Could you check a few things on this model? Use its own coordinates, in mm. A direction names the side the tool comes from. Give positions to 0.01 mm unless a question says otherwise; leave off trailing zeros. Loops run counter-clockwise (first coordinate to the right, second up) from the corner with the lowest first, then second, coordinate; pieces in that order, holes last. Notation, with made-up numbers: (58.25, 53) - (86.25, 53) arc R9 ccw to (86.25, 58) - close; hole circle Ø8 at (-38, 79.25). An arc over 180 degrees is marked (long way). Use CSV: the item, a comma, the result in double quotes.
Autodesk Inventor part; units mm, degrees
ref_plane "YZ Plane" through (0, 0, 0) normal (1, 0, 0) x (0, 1, 0)
ref_plane "XZ Plane" through (0, 0, 0) normal (0, 1, 0) x (-1, 0, 0)
ref_plane "XY Plane" through (0, 0, 0) normal (0, 0, 1) x (1, 0, 0)
sketch "main" plane through (0, 0, 0) normal (0, 0, 1) x (1, 0, 0)
  circle A0 centre (20.1733, 30.7236) radius 2.0955
  arc A1 (-24.2767, -13.7264) -> (-5.2267, 5.3236) centre (-24.2767, 5.3236) ccw
  line L0 (-5.2267, 14.8486) -> (-5.2267, 5.3236)
  line L1 (0.4529, -22.9162) -> (25.8529, 27.8838)
  arc A2 (-5.2267, 14.8486) -> (-14.7517, 24.3736) centre (-14.7517, 14.8486) ccw
  line L2 (-17.9267, 24.3736) -> (-14.7517, 24.3736)
  arc A3 (25.8529, 27.8838) -> (20.1733, 37.0736) centre (20.1733, 30.7236) ccw
  line L3 (20.1733, 37.0736) -> (-17.9267, 37.0736)
  line L4 (-30.6267, -13.7264) -> (-24.2767, -13.7264)
  circle A4 centre (-5.2267, -20.0764) radius 2.1844
  arc A5 (-5.2267, -26.4264) -> (0.4529, -22.9162) centre (-5.2267, -20.0764) ccw
  line L5 (-5.2267, -26.4264) -> (-30.6267, -26.4264)
  line L6 (-5.2267, -26.4264) -> (-30.6267, -26.4264)
  circle A6 centre (-30.6267, -20.0764) radius 2.1844
  arc A7 (-30.6267, -13.7264) -> (-30.6267, -26.4264) centre (-30.6267, -20.0764) ccw
  circle A8 centre (-5.2267, 30.7236) radius 2.1844
  circle A9 centre (7.4733, 5.3236) radius 2.0955
  arc A10 (-17.9267, 37.0736) -> (-17.9267, 24.3736) centre (-17.9267, 30.7236) ccw
  circle A11 centre (-17.9267, 30.7236) radius 2.1844
  point P0 (-10.623, 1.8831)
  point P1 (-5.2267, -13.7264)
  dimension "d0" = 12.7
  dimension "d1" = 12.7
  dimension "d2" = 4.3688
  dimension "d3" = 19.05
  dimension "d4" = 9.525
  dimension "d7" = 4.3688
  dimension "d8" = 4.191
  dimension "d10" = 4.191
sketch "Sketch1" plane through (0, 0, 0) normal (0, 0, 1) x (1, 0, 0)
  circle A0 centre (50.8, 0) radius 2.0955
  arc A1 (6.35, -44.45) -> (25.4, -25.4) centre (6.35, -25.4) ccw
  line L0 (25.4, -15.875) -> (25.4, -25.4)
  line L1 (31.0796, -53.6398) -> (56.4796, -2.8398)
  arc A2 (25.4, -15.875) -> (15.875, -6.35) centre (15.875, -15.875) ccw
  line L2 (12.7, -6.35) -> (15.875, -6.35)
  arc A3 (56.4796, -2.8398) -> (50.8, 6.35) centre (50.8, 0) ccw
  line L3 (50.8, 6.35) -> (12.7, 6.35)
  line L4 (0, -44.45) -> (6.35, -44.45)
  circle A4 centre (25.4, -50.8) radius 2.1844
  arc A5 (25.4, -57.15) -> (31.0796, -53.6398) centre (25.4, -50.8) ccw
  line L5 (25.4, -57.15) -> (0, -57.15)
  line L6 (25.4, -57.15) -> (0, -57.15)
  circle A6 centre (0, -50.8) radius 2.1844
  arc A7 (0, -44.45) -> (0, -57.15) centre (0, -50.8) ccw
  circle A8 centre (25.4, 0) radius 2.1844
  circle A9 centre (38.1, -25.4) radius 2.0955
  arc A10 (12.7, 6.35) -> (12.7, -6.35) centre (12.7, 0) ccw
  circle A11 centre (12.7, 0) radius 2.1844
  point P0 (0, 0)
extrude "Extrusion1" add sketch "Sketch1" along normal blind 1.5875
properties part number "gusset" material "Acetal Resin, White"
1) Which directions (+Z, -Z, +X, -X, +Y, -Y) give clear straight access to the entire face, cutting with the end or side of a thin tool? Please do faces 5 (the flat face through (25.4, -21, 1)), 6 (the flat face through (32, 6.35, 1)).
Answer below:
face 5,"+Z, -Z, -X"
face 6,"+Z, -Z, +X, -X, +Y"
2) We'd pull the mould along Y, two halves only. Please class faces 1 (the cylindrical face through (6.35, -0.14, 0.78)), 2 (the flat face through (13, -57.15, 1)), 3 (the flat face through (3, -44.45, 1)), 4 (the cylindrical face through (10.518, -0.096, 0.783)): +Y half, -Y half, draft (parallel to the pull), parting line (faces both ways), or undercut.
Answer below:
face 1,"undercut"
face 2,"-Y half"
face 3,"+Y half"
face 4,"undercut"
3) I need wall thicknesses on line 1 along X through (y, z) = (-1, 0.45); line 2 along X through (y, z) = (-51.5, 0.85); line 3 along Y through (x, z) = (12.7, 0.7). Which ranges of each line are inside material? Lowest first, please.
Answer below:
line 1,"x = 6.43 to 10.76, 14.64 to 23.46, 27.34 to 48.96, 52.64 to 57.07"
line 2,"x = -6.31 to -2.07, 2.07 to 23.33, 27.47 to 32.15"
line 3,"y = -57.15 to -43.36, -6.35 to -2.18, 2.18 to 6.35"
4) I'm going to push flat-ended pins straight in: P1, Ø4, axis at x = 0, y = -50.8, coming from the +Z side; P2, Ø0.5, axis at x = 2.5, z = 0.5, coming from the +Y side. Where does each tip first touch, or does it pass through?
Answer below:
P1,"passes through"
P2,"stops at y = -44.45"
5) Suppose I cut it at B-B (x = 14). Please give me the cut outline in (y, z), plus the area to 3 significant figures.
Answer below:
outline,"(-57.15, 0) - (-42.85, 0) - (-42.85, 1.59) - (-57.15, 1.59) - close; (-6.35, 0) - (-1.76, 0) - (-1.76, 1.59) - (-6.35, 1.59) - close; (1.76, 0) - (6.35, 0) - (6.35, 1.59) - (1.76, 1.59) - close"
area,"37.3 mm2"
6) Suppose I cut it at A-A (y = 0). Please give me the cut outline in (x, z).
Answer below:
outline,"(6.35, 0) - (10.52, 0) - (10.52, 1.59) - (6.35, 1.59) - close; (14.88, 0) - (23.22, 0) - (23.22, 1.59) - (14.88, 1.59) - close; (27.58, 0) - (48.7, 0) - (48.7, 1.59) - (27.58, 1.59) - close; (52.9, 0) - (57.15, 0) - (57.15, 1.59) - (52.9, 1.59) - close"
7) Suppose I cut it at D-D (x = 38.1). Please give me the cut outline in (y, z), plus the area to 3 significant figures.
Answer below:
outline,"(-39.6, 0) - (-27.5, 0) - (-27.5, 1.59) - (-39.6, 1.59) - close; (-23.3, 0) - (6.35, 0) - (6.35, 1.59) - (-23.3, 1.59) - close"
area,"66.3 mm2"
8) Suppose I cut it at C-C (z = 0.9). State how many separate pieces and enclosed holes the cut face has, plus the area to 3 significant figures.
Answer below:
separate pieces,"1"
enclosed holes,"6"
area,"1,850 mm2"
